from build123d import *

# Parameters (mm, degrees)
IZIM1_W                     = 102
IZIM1_H                     = 102
Y_KSEKLIK_EKSTR_ZYON1_DEPTH = 10
IZIM4_R                     = 2.5
KES_EKSTR_ZYON1_DEPTH       = 9.5
IZIM5_R                     = 1.5
KES_EKSTR_ZYON2_DEPTH       = 58
IZIM6_R                     = 3.5
KES_EKSTR_ZYON9_DEPTH       = 5
IZIM9_R                     = 2
KES_EKSTR_ZYON10_DEPTH      = 5
IZIM10_R                    = 1.5
KES_EKSTR_ZYON18_DEPTH      = 8
PAH1_SIZE                   = 1


with BuildPart() as part:
    # Çizim1 → Yükseklik-Ekstrüzyon1 (new body)
    with BuildSketch(Plane(origin=(0, 0, 0), x_dir=(1, 0, 0), z_dir=(0, 1, 0))):
        Rectangle(IZIM1_W, IZIM1_H)
    extrude(amount=Y_KSEKLIK_EKSTR_ZYON1_DEPTH)

    # Çizim4 → Kes-Ekstrüzyon1 (cut)
    with BuildSketch(Plane.ZY.offset(51)):
        with Locations((-8, 5)):
            Circle(IZIM4_R)
        with Locations((8, 5)):
            Circle(IZIM4_R)
    extrude(amount=-KES_EKSTR_ZYON1_DEPTH, mode=Mode.SUBTRACT)

    # Çizim5 → Kes-Ekstrüzyon2 (cut)
    with BuildSketch(Plane.ZY.offset(41.5)):
        with Locations((-8, 5)):
            Circle(IZIM5_R)
        with Locations((8, 5)):
            Circle(IZIM5_R)
    extrude(amount=-KES_EKSTR_ZYON2_DEPTH, mode=Mode.SUBTRACT)

    # Çizim6 → Kes-Ekstrüzyon9 (cut)
    with BuildSketch(Plane(origin=(0, 0, 0), x_dir=(-1, 0, 0), z_dir=(0, -1, 0))):
        with Locations(Location((33.5, -22, 0), (0, 0, 90))):
            Circle(IZIM6_R)
        with Locations(Location((33.5, 22, 0), (0, 0, 90))):
            Circle(IZIM6_R)
        with Locations(Location((-1.5, 0, 0), (0, 0, 90))):
            Circle(IZIM6_R)
        with Locations(Location((-26.5, 0, 0), (0, 0, 90))):
            Circle(IZIM6_R)
    extrude(amount=-KES_EKSTR_ZYON9_DEPTH, mode=Mode.SUBTRACT)

    # Çizim9 → Kes-Ekstrüzyon10 (cut)
    with BuildSketch(Plane.XZ.offset(-5)):
        with Locations(Location((-33.5, 22, 0), (0, 0, 270))):
            Circle(IZIM9_R)
        with Locations(Location((1.5, 0, 0), (0, 0, 270))):
            Circle(IZIM9_R)
        with Locations(Location((26.5, 0, 0), (0, 0, 270))):
            Circle(IZIM9_R)
        with Locations(Location((-33.5, -22, 0), (0, 0, 270))):
            Circle(IZIM9_R)
    extrude(amount=-KES_EKSTR_ZYON10_DEPTH, mode=Mode.SUBTRACT)

    # Çizim10 → Kes-Ekstrüzyon18 (cut)
    with BuildSketch(Plane(origin=(0, 10, 0), x_dir=(1, 0, 0), z_dir=(0, 1, 0))):
        with Locations(Location((-33.5, 8, 0), (0, 0, 270))):
            Circle(IZIM10_R)
        with Locations(Location((-33.5, -8, 0), (0, 0, 90))):
            Circle(IZIM10_R)
        with Locations(Location((14, 8, 0), (0, 0, 270))):
            Circle(IZIM10_R)
        with Locations(Location((14, -8, 0), (0, 0, 270))):
            Circle(IZIM10_R)
    extrude(amount=-KES_EKSTR_ZYON18_DEPTH, mode=Mode.SUBTRACT)

    # Pah1
    pah1_edges = [part.edges().sort_by_distance(p)[0] for p in [
        (-51, 10, 0),
        (0, 10, 51),
        (51, 10, 0),
        (0, 10, -51),
    ]]
    chamfer(pah1_edges, length=PAH1_SIZE)


solid = part.part
Source: CAD feature listing. Evaluate the final solid. Frame: model axes, mm. A direction names the side the tool comes from. Coordinates: 2 decimals unless noted, no trailing zeros. Write each loop counter-clockwise with the first axis right and the second up, starting at its lowest first coordinate (ties: lowest second). Pieces come first, ordered by that corner, then holes. Notation, with made-up numbers: M 83.25,69.5 L 114.25,69.5 A18 cw 114.25,103.5 Z; hole C -26.5,31 d2. An arc over 180 degrees is marked long. Use a Markdown table: item, result.
1) Ray query, L1, parallel to Z at x = -19.5, y = 5; L2, parallel to Z at x = -44.5, y = 6.25; L3, parallel to Z at x = -36, y = 4.75. Return the intervals inside material, ascending.
Conclusion:
| item | result |
|---|---|
| L1 | z = -51 to -9.5, -6.5 to 6.5, 9.5 to 51 |
| L2 | z = -51 to -10.17, -5.83 to 5.83, 10.17 to 51 |
| L3 | z = -51 to -24.45, -19.55 to -9.48, -6.52 to 6.52, 9.48 to 19.55, 24.45 to 51 |
2) Section C-C, the plane z = 8. Give the number of separate pieces and of enclosed holes in the cut face, then the cut area to 4 significant figures.
Conclusion:
| item | result |
|---|---|
| separate pieces | 3 |
| enclosed holes | 0 |
| area | 767.5 mm^2 |
3) Section B-B, the plane z = 22. Output: boundary loops of the cut face in (x, y), then the cut area to 3 significant figures.
Conclusion:
| item | result |
|---|---|
| outline | M -51,0 L -37,0 L -37,5 L -35.5,5 L -35.5,10 L -50,10 L -51,9 Z; M -31.5,5 L -30,5 L -30,0 L 51,0 L 51,9 L 50,10 L -31.5,10 Z |
| area | 964 mm^2 |
4) Reachability of faces 1 (the cylindrical face through (5, 2, 0)), 2 (the cylindrical face through (-35.452, 7.465, -21.566)), 3 (the cylindrical face through (13.1, 3.2, 6.8)), 4 (the cylindrical face through (-37.556, 6.265, 8.806)) from +Z, -Z, +X, -X, +Y, -Y: full face, straight path, thin tool, end or side. Return the list, or none.
Conclusion:
| item | result |
|---|---|
| face 1 | -Y |
| face 2 | +Y, -Y |
| face 3 | +Y |
| face 4 | -X |
5) Mould query, pull axis X, two halves, no side actions, for faces 5 (the flat face through (25, 5, -2)), 6 (the cylindrical face through (-10.1, 4.1, 6.8)), 7 (the flat face through (-41.5, 3, 8)). Classes: pulls with the +X half, pulls with the -X half, needs draft (parallel to the pull), parting line crosses it, or undercut.
Conclusion:
| item | result |
|---|---|
| face 5 | undercut |
| face 6 | needs draft |
| face 7 | pulls with the -X half |
6) First-contact query: pin 1 Ø8 at (x, z) = (-33.5, -22) entering from -Y; pin 2 Ø1.5 at (y, z) = (5, 7.5) entering from -X; pin 3 Ø1.5 at (x, z) = (13.5, -8) entering from +Y; pin 4 Ø2 at (x, z) = (2, -0.5) entering from -Y. Flat tips, straight axial feed; report the tip coordinate or a pass-through.
Conclusion:
| item | result |
|---|---|
| pin 1 | stops at y = 0 |
| pin 2 | stops at x = 16.5 |
| pin 3 | stops at y = 2 |
| pin 4 | passes through |
7) Section A-A, the plane x = 1.5. Output: boundary loops of the cut face in (y, z).
Conclusion:
| item | result |
|---|---|
| outline | M 0,-51 L 9,-51 L 10,-50 L 10,-2 L 5,-2 L 5,-3.5 L 0,-3.5 Z; M 0,3.5 L 5,3.5 L 5,2 L 10,2 L 10,50 L 9,51 L 0,51 Z; hole C 5,-8 d3; hole C 5,8 d3 |
